The listing builds one solid part. Answer for the finished solid, in the listing's coordinates (mm). A direction names the side the tool comes from. Give positions to 0.01 mm unless a question says otherwise; leave off trailing zeros. Loops run counter-clockwise (first coordinate to the right, second up) from the corner with the lowest first, then second, coordinate; pieces in that order, holes last.
Item 1: Section A-A, the plane z = 22 is taken. Give the vertices of the cut face in (x, y), and give its area (3 significant figures).
Item 2: The mould has two halves that part along Z. Classify faces 4 (the face through (28.092, 20.601, -5.07)), 5 (the face through (0, 0, 30)), 6 (the face through (11.5, 0.13, 20.69)): pulls with the +Z half, pulls with the -Z half, needs draft (parallel to the pull), parting line crosses it, or undercut.
Item 3: Section D-D, the plane y = 0 is taken. Give the vertices of the cut face in (x, z), and give its area (3 significant figures).
Item 4: Section B-B, the plane x = 0 is taken. Give the vertices of the cut face in (y, z).
Item 5: Section C-C, the plane z = 10 is taken. Give the vertices of the cut face in (x, y).
Item 6: Each of these flat-tipped pins is pushed along its axis until it touches: pin 1 Ø3 at (x, z) = (-3, 22) entering from -Y; pin 2 Ø3 at (x, z) = (8, -1) entering from +Y; pin 3 Ø5.5 at (x, z) = (0, 10) entering from +Y. Where does it stop, or does it pass through?
Item 7: A tool of negligible diameter and unlimited length cuts with its end or side. For faces 1 (the face through (17.5, 0, 15)), 2 (the face through (26.8, 13.66, -4.93)), 3 (the face through (0, 9.5, 15)), from which of +Z, -Z, +X, -X, +Y, -Y can it reach the whole face along a straight path? Write none if from no direction.
Item 8: Consider line 1 along X through (y, z) = (-4.75, 22); line 2 along Y through (x, z) = (30, -5.75); line 3 along Z through (x, y) = (4, 19). Determine where each line is inside the solid, lowest interval first.
from build123d import *

# Parameters (mm, degrees)
BASE_FLANGE1_DEPTH        = 10
F_4_0MM_DOWEL_HOLE1_D     = 4
F_4_0MM_DOWEL_HOLE1_DEPTH = 16
F_4_0MM_DOWEL_HOLE1_TIP   = 1.201721238
FILLET1_R                 = 5
F_4_0MM_DOWEL_HOLE2_D     = 4
F_4_0MM_DOWEL_HOLE2_DEPTH = 16
F_4_0MM_DOWEL_HOLE2_TIP   = 1.201721238
SKETCH17_W                = 35
SKETCH17_H                = 19
BOSS_EXTRUDE1_DEPTH       = 30
SKETCH18_R                = 1.65
CUT_EXTRUDE1_DEPTH        = 56.778580118
FILLET2_R                 = 1


# Sheet-metal steps are written as plain solids
with BuildPart() as part:
    # Sketch1 → Base-Flange1 (new body)
    with BuildSketch(Plane.XY):
        with BuildLine():
            Line((14.442758409, 13.834982094), (28.058549313, 22.91217603))
            ThreePointArc((28.058549313, 22.91217603), (32.91217603, 21.941450687), (31.941450687, 17.08782397))
            Line((31.941450687, 17.08782397), (18.325659783, 8.010630034))
            ThreePointArc((18.325659783, 8.010630034), (20, 0), (18.325659783, -8.010630034))
            Line((18.325659783, -8.010630034), (31.941450687, -17.08782397))
            ThreePointArc((31.941450687, -17.08782397), (32.91217603, -21.941450687), (28.058549313, -22.91217603))
            Line((28.058549313, -22.91217603), (14.442758409, -13.834982094))
            ThreePointArc((14.442758409, -13.834982094), (0, -20), (-14.442758409, -13.834982094))
            Line((-14.442758409, -13.834982094), (-28.058549313, -22.91217603))
            ThreePointArc((-28.058549313, -22.91217603), (-32.91217603, -21.941450687), (-31.941450687, -17.08782397))
            Line((-31.941450687, -17.08782397), (-18.325659783, -8.010630034))
            ThreePointArc((-18.325659783, -8.010630034), (-20, 0), (-18.325659783, 8.010630034))
            Line((-18.325659783, 8.010630034), (-31.941450687, 17.08782397))
            ThreePointArc((-31.941450687, 17.08782397), (-32.91217603, 21.941450687), (-28.058549313, 22.91217603))
            Line((-28.058549313, 22.91217603), (-14.442758409, 13.834982094))
            ThreePointArc((-14.442758409, 13.834982094), (0, 20), (14.442758409, 13.834982094))
        make_face()
    extrude(amount=-BASE_FLANGE1_DEPTH)

    # Ø4.0mm Dowel Hole1
    with Locations(Plane.XY):
        with Locations((-30, 20), (30, -20), (-30, -20), (30, 20)):
            Hole(F_4_0MM_DOWEL_HOLE1_D / 2, depth=F_4_0MM_DOWEL_HOLE1_DEPTH)
            with Locations((0, 0, -(F_4_0MM_DOWEL_HOLE1_DEPTH + F_4_0MM_DOWEL_HOLE1_TIP / 2))):  # 118° drill point
                Cone(0, F_4_0MM_DOWEL_HOLE1_D / 2, F_4_0MM_DOWEL_HOLE1_TIP, mode=Mode.SUBTRACT)

    # Fillet1
    fillet1_edges = [part.edges().sort_by_distance(p)[0] for p in [
        (18.325659783, 8.010630034, -5),
        (18.325659783, -8.010630034, -5),
        (14.442758409, -13.834982094, -5),
        (-14.442758409, -13.834982094, -5),
        (-18.325659783, -8.010630034, -5),
        (-18.325659783, 8.010630034, -5),
        (-14.442758409, 13.834982094, -5),
        (14.442758409, 13.834982094, -5),
    ]]
    fillet(fillet1_edges, radius=FILLET1_R)

    # Ø4.0mm Dowel Hole2
    with Locations(Plane(origin=(0, 0, -10), x_dir=(-1, 0, 0), z_dir=(0, 0, -1))):
        with Locations((0, 0)):
            Hole(F_4_0MM_DOWEL_HOLE2_D / 2, depth=F_4_0MM_DOWEL_HOLE2_DEPTH)
            with Locations((0, 0, -(F_4_0MM_DOWEL_HOLE2_DEPTH + F_4_0MM_DOWEL_HOLE2_TIP / 2))):  # 118° drill point
                Cone(0, F_4_0MM_DOWEL_HOLE2_D / 2, F_4_0MM_DOWEL_HOLE2_TIP, mode=Mode.SUBTRACT)

    # Sketch17 → Boss-Extrude1 (add)
    with BuildSketch(Plane.XY):
        Rectangle(SKETCH17_W, SKETCH17_H)
    extrude(amount=BOSS_EXTRUDE1_DEPTH)

    # Sketch18 → Cut-Extrude1 (cut, through all)
    with BuildSketch(Plane(origin=(0, 9.5, 0), x_dir=(1, 0, 0), z_dir=(0, 1, 0))):
        with Locations(Location((0, -10, 0), (0, 0, 270))):
            Circle(SKETCH18_R)
        with Locations(Location((-12.5, -22, 0), (0, 0, 270))):
            Circle(SKETCH18_R)
        with Locations(Location((12.5, -22, 0), (0, 0, 270))):
            Circle(SKETCH18_R)
    extrude(amount=-CUT_EXTRUDE1_DEPTH, mode=Mode.SUBTRACT)

    # Fillet2
    fillet2_edges = [part.edges().sort_by_distance(p)[0] for p in [
        (17.5, 0, 0),
        (17.5, -9.5, 15),
        (0, 9.5, 0),
        (17.5, 9.5, 15),
        (-17.5, 0, 0),
        (-17.5, 9.5, 15),
        (0, -9.5, 0),
        (-17.5, -9.5, 15),
    ]]
    fillet(fillet2_edges, radius=FILLET2_R)


solid = part.part
Worked answers:
1. outline: (-17.5, -8.5) arc R1 ccw to (-16.5, -9.5) - (-14.15, -9.5) - (-14.15, 9.5) - (-16.5, 9.5) arc R1 ccw to (-17.5, 8.5) - close; (-10.85, -9.5) - (10.85, -9.5) - (10.85, 9.5) - (-10.85, 9.5) - close; (14.15, -9.5) - (16.5, -9.5) arc R1 ccw to (17.5, -8.5) - (17.5, 8.5) arc R1 ccw to (16.5, 9.5) - (14.15, 9.5) - close
1. area: 539 mm2
2. face 4: needs draft
2. face 5: pulls with the +Z half
2. face 6: undercut
3. outline: (-20, -10) - (-2, -10) - (-2, 0) - (2, 0) - (2, -10) - (20, -10) - (20, 0) - (18.5, 0) arc R1 cw to (17.5, 1) - (17.5, 30) - (-17.5, 30) - (-17.5, 1) arc R1 cw to (-18.5, 0) - (-20, 0) - close; hole circle Ø3.3 at (-12.5, 22); hole circle Ø3.3 at (0, 10); hole circle Ø3.3 at (12.5, 22)
3. area: 1,380 mm2
4. outline: (-20, -10) - (-2, -10) - (-2, 0) - (2, 0) - (2, -10) - (20, -10) - (20, 0) - (10.5, 0) arc R1 cw to (9.5, 1) - (9.5, 8.35) - (-9.5, 8.35) - (-9.5, 1) arc R1 cw to (-10.5, 0) - (-20, 0) - close; (-9.5, 11.65) - (9.5, 11.65) - (9.5, 30) - (-9.5, 30) - close
5. outline: (-17.5, -8.5) arc R1 ccw to (-16.5, -9.5) - (-1.65, -9.5) - (-1.65, 9.5) - (-16.5, 9.5) arc R1 ccw to (-17.5, 8.5) - close; (1.65, -9.5) - (16.5, -9.5) arc R1 ccw to (17.5, -8.5) - (17.5, 8.5) arc R1 ccw to (16.5, 9.5) - (1.65, 9.5) - close
6. pin 1: stops at y = -9.5
6. pin 2: stops at y = 18.91
6. pin 3: stops at y = 9.5
7. face 1: +Z, +X, +Y, -Y
7. face 2: +Z, -Z, +X
7. face 3: +Z, +X, -X, +Y
8. line 1: x = -17.5 to -14.15, -10.85 to 10.85, 14.15 to 17.5
8. line 2: y = -23.5 to -22, -18 to -15.79, 15.79 to 18, 22 to 23.5
8. line 3: z = -10 to 0
